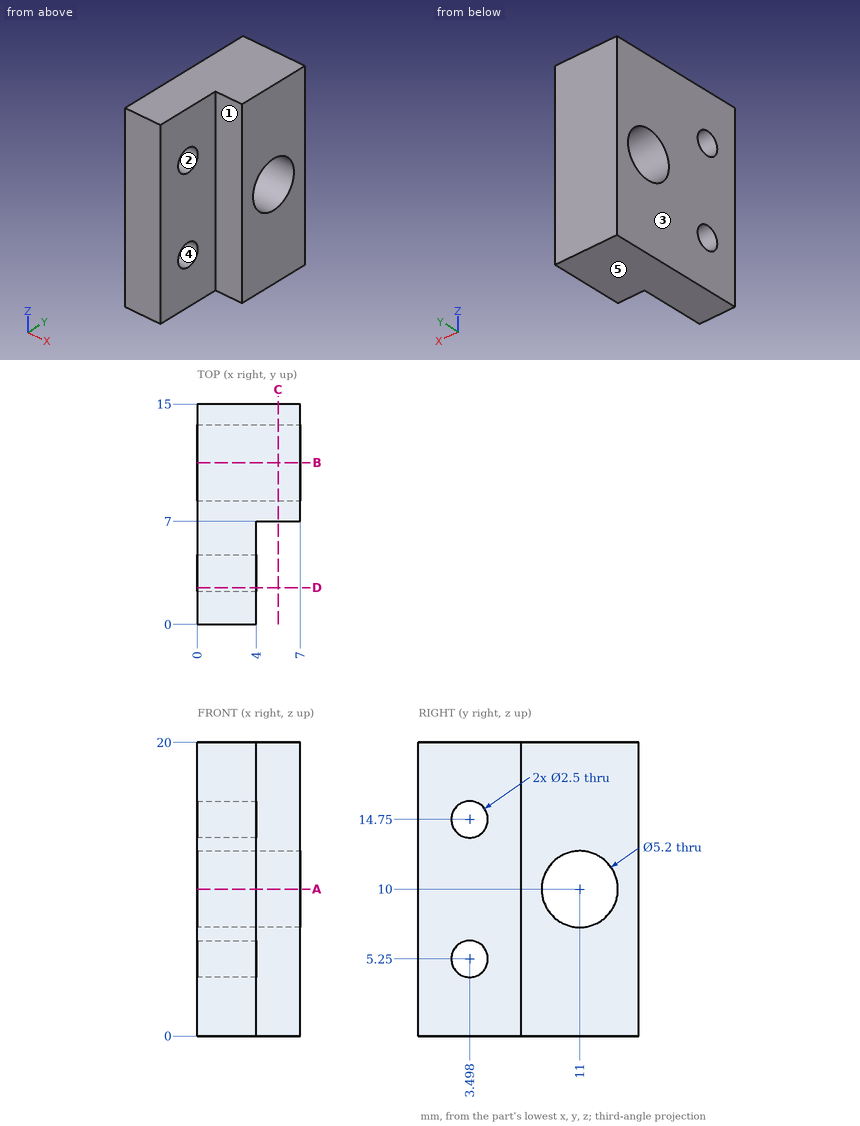
Geometry check sheet. Reference: drawing and pictorial views, mm from the part's lowest x, y, z. A direction names the side the tool comes from. Give positions to 0.01 mm unless a question says otherwise; leave off trailing zeros. Order: outer loops, then holes, each group sorted by start corner. A loop starts at its lowest first (then second) coordinate and runs counter-clockwise, first axis right, second up.
1. Gauge pin test, flat ends, axial feed: pin 1 Ø2 at (y, z) = (3.5, 14.75) entering from +X; pin 2 Ø2.5 at (x, z) = (6, 9.5) entering from -Y; pin 3 Ø7.5 at (y, z) = (3, 6.5) entering from +X. Record the tip position at first contact, or that the pin passes through.
2. Section check D-D, the plane y = 2.5. Enter the section's corners in (x, z).
3. Release check for a two-part mould opening along Z. For the marked faces 3, 4 and 5 record: pulls with the +Z half, pulls with the -Z half, needs draft (parallel to the pull), parting line crosses it, or undercut.
4. Section check B-B, the plane y = 11. Enter the section's corners in (x, z), and give its area (3 significant figures).
5. Section check C-C, the plane x = 5.5. Enter the section's corners in (y, z), and give its area (3 significant figures).
6. Access from +Z, -Z, +X, -X, +Y, -Y to the whole of each face (thin tool, end or side, straight path). Record for the marked faces 1 and 2.
7. Thickness scan on L1, parallel to Y at x = 3.15, z = 14.75; L2, parallel to Y at x = 1.5, z = 10; L3, parallel to Z at x = 3.75, y = 9.5. Record the ranges inside material, lowest first.
8. Section check A-A, the plane z = 10. Enter the section's corners in (x, y).
Values follow:
1. pin 1: passes through
1. pin 2: stops at y = 7
1. pin 3: stops at x = 4
2. outline: (0, 0) - (4, 0) - (4, 4.5) - (0, 4.5) - close; (0, 6) - (4, 6) - (4, 14) - (0, 14) - close; (0, 15.5) - (4, 15.5) - (4, 20) - (0, 20) - close
3. face 3: needs draft
3. face 4: undercut
3. face 5: pulls with the -Z half
4. outline: (0, 0) - (7, 0) - (7, 7.4) - (0, 7.4) - close; (0, 12.6) - (7, 12.6) - (7, 20) - (0, 20) - close
4. area: 104 mm2
5. outline: (7, 0) - (15, 0) - (15, 20) - (7, 20) - close; hole circle Ø5.2 at (11, 10)
5. area: 139 mm2
6. face 1: +Z, -Z, +X, -Y
6. face 2: +X, -X
7. L1: y = 0 to 2.25, 4.75 to 15
7. L2: y = 0 to 8.4, 13.6 to 15
7. L3: z = 0 to 7.88, 12.12 to 20
8. outline: (0, 0) - (4, 0) - (4, 7) - (7, 7) - (7, 8.4) - (0, 8.4) - close; (0, 13.6) - (7, 13.6) - (7, 15) - (0, 15) - close
